Work out the finished part from the listing and answer in its coordinate system (mm). Face numbers are marked on the shaded views. A direction names the side the tool comes from. Coordinates: 2 decimals unless noted, no trailing zeros. Order: outer loops, then holes, each group sorted by start corner. A loop starts at its lowest first (then second) coordinate and runs counter-clockwise, first axis right, second up. Notation, with made-up numbers: M 21.5,54 L 27.5,54 A17 cw 27.5,58 Z; hole C 58.5,78 d2. An arc over 180 degrees is marked long. Answer in a Markdown table with one row per item. Add a question column.
Item 1: The part is cut by section C-C (y = 0). Write down the section's boundary in (x, z), then the cut area to 3 significant figures.
Item 2: The part is cut by section A-A (x = 0). Write down the section's boundary in (y, z) (3 decimals).
Item 3: Consider line 1 (Z direction, x = 0, y = 1); line 2 (X direction, y = 3.5, z = 0). Determine where each line is inside the solid, lowest interval first. Write a range as from..to.
Item 4: The part is cut by section B-B (z = 0). Write down the section's boundary in (x, y) (3 decimals).
Item 5: Flat-ended cylindrical pins translate along their axes: pin 1 Ø7 at (x, z) = (0, 0) entering from -Y; pin 2 Ø4 at (x, z) = (0, -8) entering from -Y (3 decimals); pin 3 Ø1 at (y, z) = (-4.5, 1.5) entering from +X; pin 4 Ø4 at (x, z) = (8, 0) entering from +Y (3 decimals). Find the tip coordinate at first contact, or state that the pin passes through.
Item 6: Which of the six approach directions +Z, -Z, +X, -X, +Y, -Y give full straight-line access (tool end or side, diameter ignored) to the marked faces 4 and 5?
Item 7: The part is cut by section D-D (x = -9.25). Write down the section's boundary in (y, z) (3 decimals), then the cut area to 3 significant figures.
Item 8: The mould has two halves that part along Z. Classify the marked faces 1, 2 and 3: released by +Z, released by -Z, zero draft, split by the parting line, or undercut.
from build123d import *

# Parameters (mm, degrees)
SKETCH1_R           = 4.699
SKETCH1_R_2         = 3
BOSS_EXTRUDE1_DEPTH = 6.35
SKETCH1_3_R         = 11.049
SKETCH1_3_R_2       = 1.63195
SKETCH1_3_R_3       = 4.699
BOSS_EXTRUDE2_DEPTH = 3.175


with BuildPart() as part:
    # Sketch1 → Boss-Extrude1 (new, symmetric)
    with BuildSketch(Plane(origin=(0, 0, 0), x_dir=(1, 0, 0), z_dir=(0, 1, 0))):
        Circle(SKETCH1_R)
        Circle(SKETCH1_R_2, mode=Mode.SUBTRACT)
    extrude(amount=BOSS_EXTRUDE1_DEPTH, both=True)

    # Sketch1<3> → Boss-Extrude2 (add, symmetric)
    with BuildSketch(Plane(origin=(0, 0, 0), x_dir=(1, 0, 0), z_dir=(0, 1, 0))):
        Circle(SKETCH1_3_R)
        with Locations((-8, 0)):
            Circle(SKETCH1_3_R_2, mode=Mode.SUBTRACT)
        Circle(SKETCH1_3_R_3, mode=Mode.SUBTRACT)
        with Locations((0, -8)):
            Circle(SKETCH1_3_R_2, mode=Mode.SUBTRACT)
        with Locations((0, 8)):
            Circle(SKETCH1_3_R_2, mode=Mode.SUBTRACT)
        with Locations((8, 0)):
            Circle(SKETCH1_3_R_2, mode=Mode.SUBTRACT)
    extrude(amount=BOSS_EXTRUDE2_DEPTH, both=True)


solid = part.part
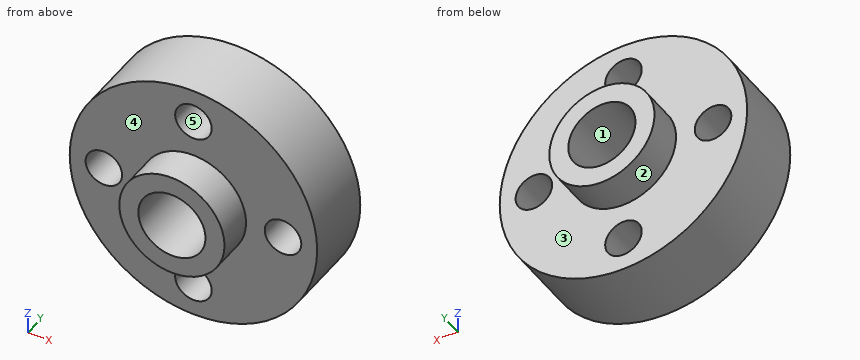
Reply:
| question | item | result |
|---|---|---|
| 1 | outline | C 0,0 d22.1; hole C -8,0 d3.26; hole C 0,0 d6; hole C 0,-8 d3.26; hole C 0,8 d3.26; hole C 8,0 d3.26 |
| 1 | area | 322 mm2 |
| 2 | outline | M -6.35,-4.699 L -3.175,-4.699 L -3.175,-6.368 L 3.175,-6.368 L 3.175,-4.699 L 6.35,-4.699 L 6.35,-3 L -6.35,-3 Z; M -6.35,3 L 6.35,3 L 6.35,4.699 L 3.175,4.699 L 3.175,6.368 L -3.175,6.368 L -3.175,4.699 L -6.35,4.699 Z; M -3.175,-11.049 L 3.175,-11.049 L 3.175,-9.632 L -3.175,-9.632 Z; M -3.175,9.632 L 3.175,9.632 L 3.175,11.049 L -3.175,11.049 Z |
| 3 | line 1 | z = -11.05..-9.63, -6.37..-3, 3..6.37, 9.63..11.05 |
| 3 | line 2 | x = -4.7..-3, 3..4.7 |
| 4 | outline | M -11.049,-3.175 L -9.632,-3.175 L -9.632,3.175 L -11.049,3.175 Z; M -6.368,-3.175 L -4.699,-3.175 L -4.699,-6.35 L -3,-6.35 L -3,6.35 L -4.699,6.35 L -4.699,3.175 L -6.368,3.175 Z; M 3,-6.35 L 4.699,-6.35 L 4.699,-3.175 L 6.368,-3.175 L 6.368,3.175 L 4.699,3.175 L 4.699,6.35 L 3,6.35 Z; M 9.632,-3.175 L 11.049,-3.175 L 11.049,3.175 L 9.632,3.175 Z |
| 5 | pin 1 | stops at y = -6.35 |
| 5 | pin 2 | stops at y = -3.175 |
| 5 | pin 3 | stops at x = 4.59 |
| 5 | pin 4 | stops at y = 3.175 |
| 6 | face 4 | -Y |
| 6 | face 5 | +Y, -Y |
| 7 | outline | M -3.175,-6.043 L 3.175,-6.043 L 3.175,-1.049 L -3.175,-1.049 Z; M -3.175,1.049 L 3.175,1.049 L 3.175,6.043 L -3.175,6.043 Z |
| 7 | area | 63.4 mm2 |
| 8 | face 1 | undercut |
| 8 | face 2 | split by the parting line |
| 8 | face 3 | zero draft |
